from build123d import *

# Parameters (mm, degrees)
F2_DEPTH = 25.4
F0_R     = 76.2
F3_DEPTH = 152.4
F4_DEPTH = 152.4


# Not quite as in the source:
# - an extrude ends at something that could not be found from the text; its depth is read off the source's solid


with BuildPart() as f2:
    # F1 (on Top) → F2 (new body)
    with BuildSketch(Plane.XY):
        with BuildLine():
            Line((0, 19.05), (0, 0))
            Line((0, 0), (19.05, 0))
            ThreePointArc((19.05, 0), (5.5796158184, 5.5796158184), (0, 19.05))
        make_face()
        with BuildLine():
            ThreePointArc((0, 19.05), (5.5796158184, 5.5796158184), (19.05, 0))
            Line((19.05, 0), (57.15, 0))
            ThreePointArc((57.15, 0), (70.6203841816, 5.5796158184), (76.2, 19.05))
            ThreePointArc((76.2, 19.05), (70.6203841816, 32.5203841816), (57.15, 38.1))
            Line((57.15, 38.1), (19.05, 38.1))
            ThreePointArc((19.05, 38.1), (5.5796158184, 32.5203841816), (0, 19.05))
        make_face()
        with BuildLine():
            Line((0, 38.1), (0, 19.05))
            ThreePointArc((0, 19.05), (5.5796158184, 32.5203841816), (19.05, 38.1))
            Line((19.05, 38.1), (0, 38.1))
        make_face()
        with BuildLine():
            ThreePointArc((76.2, 19.05), (70.6203841816, 5.5796158184), (57.15, 0))
            Line((57.15, 0), (76.2, 0))
            Line((76.2, 0), (76.2, 19.05))
        make_face()
        with BuildLine():
            ThreePointArc((57.15, 38.1), (70.6203841816, 32.5203841816), (76.2, 19.05))
            Line((76.2, 19.05), (76.2, 38.1))
            Line((76.2, 38.1), (57.15, 38.1))
        make_face()
    extrude(amount=F2_DEPTH)

    # F0 (on Top) → F3 (join, through all)
    with BuildSketch(Plane.XY):
        Circle(F0_R)
    extrude(amount=-F3_DEPTH)

    # F0 (on Top) → F4 (join)
    with BuildSketch(Plane.XY):
        Circle(F0_R)
    extrude(amount=-F4_DEPTH)


solid = f2.part
Geometry: final body of the model. Coordinates: model frame, mm. A direction names the side the tool comes from. Coordinates: 2 decimals unless noted, no trailing zeros. Loops run counter-clockwise (first coordinate to the right, second up) from the corner with the lowest first, then second, coordinate; pieces in that order, holes last. Notation, with made-up numbers: (57, 87) - (93, 87) arc R25 ccw to (93, 115) - close; hole circle Ø6 at (20, -17). An arc over 180 degrees is marked (long way). Put each result on its own line as item: value. Start each with the question number.
Q1. Cut plane C-C, the plane y = -19. Return loops of the section in (x, z).
Q2. Set-up query: faces 1 (the flat face through (73, 29, 0)), 2 (the flat face through (39, 38.1, 13)), 3 (the flat face through (0, 19, 13)). Return all of +Z, -Z, +X, -X, +Y, -Y with unobstructed straight access to the full face (end or side cutting, diameter ignored); none if empty.
Q3. Pin query (flat end, axial travel): pin 1 Ø12 at (y, z) = (-61, -128.5) entering from -X; pin 2 Ø5 at (y, z) = (-14.5, -6) entering from -X; pin 3 Ø7.5 at (y, z) = (18, 9.5) entering from -X. Return the tip coordinate at first contact, or that it passes through.
Q4. Cut plane B-B, the plane z = -25. Return loops of the section in (x, y).
Q5. Line query: line 1 (Z direction, x = 41, y = -42.5); line 2 (X direction, y = 2.5, z = -81); line 3 (X direction, y = 33.5, z = 11). Output: solid intervals per line, ascending.
Q6. Cut plane D-D, the plane x = 4. Return loops of the section in (y, z).
Q7. Cut plane A-A, the plane x = 44.5. Return loops of the section in (y, z), and give its area (3 significant figures).
Filled sheet:
1. outline: (-73.79, -152.4) - (73.79, -152.4) - (73.79, 0) - (-73.79, 0) - close
2. face 1: -Z, +X, +Y
2. face 2: +Z, +X, -X, +Y
2. face 3: +Z, -X, +Y, -Y
3. pin 1: x = -52.74
3. pin 2: x = -75.25
3. pin 3: x = 0
4. outline: circle Ø152.4 at (0, 0)
5. line 1: -152.4 to 0
5. line 2: -76.16 to 76.16
5. line 3: 0 to 76.2
6. outline: (-76.09, -152.4) - (76.09, -152.4) - (76.09, 0) - (38.1, 0) - (38.1, 25.4) - (0, 25.4) - (0, 0) - (-76.09, 0) - close
7. outline: (-61.86, -152.4) - (61.86, -152.4) - (61.86, 0) - (38.1, 0) - (38.1, 25.4) - (0, 25.4) - (0, 0) - (-61.86, 0) - close
7. area: 19,800 mm²
